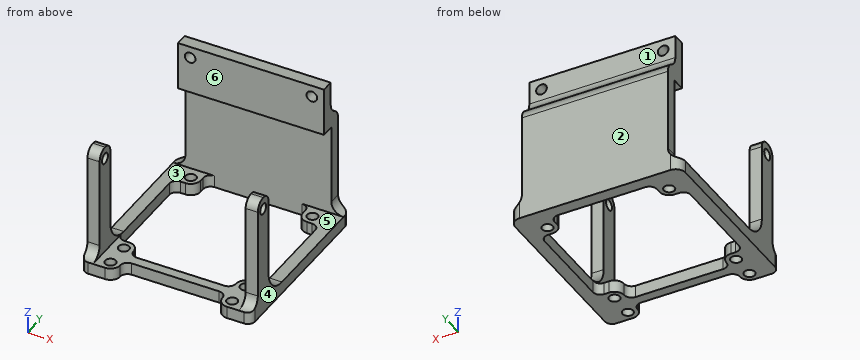
from build123d import *

# Parameters (mm, degrees)
SKETCH1_R           = 2.2
BOSS_EXTRUDE1_DEPTH = 5
FILLET1_R           = 3
FILLET2_R           = 3
SKETCH2_W           = 70
SKETCH2_H           = 43
BOSS_EXTRUDE2_DEPTH = 5
SKETCH3_W           = 70
SKETCH3_H           = 10.5
BOSS_EXTRUDE3_DEPTH = 5
SKETCH4_W           = 70
SKETCH4_H           = 5
BOSS_EXTRUDE4_DEPTH = 15
FILLET3_R           = 5.5
SKETCH6_W           = 5
SKETCH6_H           = 58
CUT_EXTRUDE1_DEPTH  = 15
FILLET4_R           = 5.5
FILLET5_R           = 5
SKETCH7_R           = 2.2
CUT_EXTRUDE2_DEPTH  = 15
SKETCH8_W           = 5
SKETCH8_H           = 8
BOSS_EXTRUDE5_DEPTH = 46
FILLET7_R           = 10
FILLET8_R           = 3
FILLET9_R           = 5
SKETCH10_R          = 2.2
CUT_EXTRUDE3_DEPTH  = 178.791001057
FILLET10_R          = 4
FILLET11_R          = 4
FILLET12_R          = 4


# Some blends are built 0.0001 mm under size
with BuildPart() as part:
    # Sketch1 → Boss-Extrude1 (new body)
    with BuildSketch(Plane.XY):
        with BuildLine():
            Line((-45.5, 87.8), (-45.5, 90.8))
            ThreePointArc((-45.5, 90.8), (-44.328427125, 93.628427125), (-41.5, 94.8))
            Line((-41.5, 94.8), (-36.5, 94.8))
            Line((-36.5, 94.8), (-36.5, 136.8))
            Line((-36.5, 136.8), (-41.5, 136.8))
            ThreePointArc((-41.5, 136.8), (-44.328427125, 137.971572875), (-45.5, 140.8))
            Line((-45.5, 140.8), (-45.5, 145.8))
            Line((-45.5, 145.8), (-36.5, 145.8))
            Line((-36.5, 145.8), (-31.5, 145.8))
            Line((-31.5, 145.8), (-31.5, 76.8))
            Line((-31.5, 76.8), (-36.5, 76.8))
            Line((-36.5, 76.8), (-41.5, 76.8))
            ThreePointArc((-41.5, 76.8), (-44.328427125, 77.971572875), (-45.5, 80.8))
            Line((-45.5, 80.8), (-45.5, 83.8))
            Line((-45.5, 83.8), (-87.5, 83.8))
            Line((-87.5, 83.8), (-87.5, 80.8))
            ThreePointArc((-87.5, 80.8), (-88.671572875, 77.971572875), (-91.5, 76.8))
            Line((-91.5, 76.8), (-96.5, 76.8))
            Line((-96.5, 76.8), (-101.5, 76.8))
            Line((-101.5, 76.8), (-101.5, 145.8))
            Line((-101.5, 145.8), (-96.5, 145.8))
            Line((-96.5, 145.8), (-87.5, 145.8))
            Line((-87.5, 145.8), (-87.5, 140.8))
            ThreePointArc((-87.5, 140.8), (-88.671572875, 137.971572875), (-91.5, 136.8))
            Line((-91.5, 136.8), (-96.5, 136.8))
            Line((-96.5, 136.8), (-96.5, 94.8))
            Line((-96.5, 94.8), (-91.5, 94.8))
            ThreePointArc((-91.5, 94.8), (-88.671572875, 93.628427125), (-87.5, 90.8))
            Line((-87.5, 90.8), (-87.5, 87.8))
            Line((-87.5, 87.8), (-45.5, 87.8))
        make_face()
        with Locations((-91.5, 140.8)):
            Circle(SKETCH1_R, mode=Mode.SUBTRACT)
        with Locations(Location((-41.5, 140.8, 0), (0, 0, 180))):
            Circle(SKETCH1_R, mode=Mode.SUBTRACT)
        with Locations((-41.5, 90.8)):
            Circle(SKETCH1_R, mode=Mode.SUBTRACT)
        with Locations(Location((-91.5, 90.8, 0), (0, 0, 180))):
            Circle(SKETCH1_R, mode=Mode.SUBTRACT)
        with Locations((-91.5, 80.8)):
            Circle(SKETCH1_R, mode=Mode.SUBTRACT)
        with Locations(Location((-41.5, 80.8, 0), (0, 0, 180))):
            Circle(SKETCH1_R, mode=Mode.SUBTRACT)
    extrude(amount=BOSS_EXTRUDE1_DEPTH)

    # Fillet1
    fillet1_edges = [part.edges().sort_by_distance(p)[0] for p in [
        (-36.5, 136.8, 2.5),
        (-96.5, 136.8, 2.5),
        (-36.5, 94.8, 2.5),
        (-45.5, 87.8, 2.5),
        (-45.5, 83.8, 2.5),
        (-87.5, 83.8, 2.5),
        (-87.5, 87.8, 2.5),
        (-96.5, 94.8, 2.5),
    ]]
    fillet(fillet1_edges, radius=FILLET1_R - 0.0001)  # a hair under: the kernel refuses the full size

    # Fillet2
    fillet2_edges = [part.edges().sort_by_distance(p)[0] for p in [
        (-31.5, 76.8, 2.5),
        (-101.5, 76.8, 2.5),
    ]]
    fillet(fillet2_edges, radius=FILLET2_R)

    # Sketch2 → Boss-Extrude2 (add)
    with BuildSketch(Plane(origin=(0, 145.8, 0), x_dir=(1, 0, 0), z_dir=(0, 1, 0))):
        with Locations((-66.5, -21.5)):
            Rectangle(SKETCH2_W, SKETCH2_H)
    extrude(amount=BOSS_EXTRUDE2_DEPTH)

    # Sketch3 → Boss-Extrude3 (add)
    with BuildSketch(Plane.XY.offset(43)):
        with Locations((-66.5, 145.55)):
            Rectangle(SKETCH3_W, SKETCH3_H)
    extrude(amount=BOSS_EXTRUDE3_DEPTH)

    # Sketch4 → Boss-Extrude4 (add)
    with BuildSketch(Plane.XY.offset(48)):
        with Locations((-66.5, 142.8)):
            Rectangle(SKETCH4_W, SKETCH4_H)
    extrude(amount=BOSS_EXTRUDE4_DEPTH)

    # Fillet3
    fillet3_edges = [part.edges().sort_by_distance(p)[0] for p in [
        (-66.5, 145.3, 48),
    ]]
    fillet(fillet3_edges, radius=FILLET3_R - 0.0001)  # a hair under: the kernel refuses the full size

    # Sketch6 → Cut-Extrude1 (cut)
    with BuildSketch(Plane(origin=(0, 150.8, 0), x_dir=(1, 0, 0), z_dir=(0, 1, 0))):
        with Locations((-99, -34)):
            Rectangle(SKETCH6_W, SKETCH6_H)
        with Locations((-34, -34)):
            Rectangle(SKETCH6_W, SKETCH6_H)
    extrude(amount=-CUT_EXTRUDE1_DEPTH, mode=Mode.SUBTRACT)

    # Fillet4
    fillet4_edges = [part.edges().sort_by_distance(p)[0] for p in [
        (-66.5, 150.8, 48),
    ]]
    fillet(fillet4_edges, radius=FILLET4_R)

    # Fillet5
    fillet5_edges = [part.edges().sort_by_distance(p)[0] for p in [
        (-36.5, 148.3, 5),
        (-96.5, 148.3, 5),
    ]]
    fillet(fillet5_edges, radius=FILLET5_R - 0.0001)  # a hair under: the kernel refuses the full size

    # Sketch7 → Cut-Extrude2 (cut)
    with BuildSketch(Plane(origin=(0, 145.3, 0), x_dir=(1, 0, 0), z_dir=(0, 1, 0))):
        with Locations(Location((-91.5, -58.25, 0), (0, 0, 270))):
            Circle(SKETCH7_R)
        with Locations(Location((-41.5, -58.25, 0), (0, 0, 270))):
            Circle(SKETCH7_R)
    extrude(amount=-CUT_EXTRUDE2_DEPTH, mode=Mode.SUBTRACT)

    # Sketch8 → Boss-Extrude5 (add)
    with BuildSketch(Plane.XY.offset(5)):
        with Locations((-99, 85.8)):
            Rectangle(SKETCH8_W, SKETCH8_H)
        with Locations((-34, 85.8)):
            Rectangle(SKETCH8_W, SKETCH8_H)
    extrude(amount=BOSS_EXTRUDE5_DEPTH)

    # Fillet7
    # the kernel refuses this fillet: 10 mm, written as the material it adds along each edge
    with BuildSketch(Plane(origin=(-101.5, 89.8, 5), x_dir=(0, 1, 0), z_dir=(1, 0, 0))) as fillet7_piece_1:
        with BuildLine():
            CenterArc((FILLET7_R, FILLET7_R), FILLET7_R, 180, 90)
            Line((0, FILLET7_R), (0, 0))
            Line((0, 0), (FILLET7_R, 0))
        make_face()
    extrude(amount=5)
    with BuildSketch(Plane(origin=(-31.5, 89.8, 5), x_dir=(0, 1, 0), z_dir=(-1, 0, 0))) as fillet7_piece_2:
        with BuildLine():
            CenterArc((FILLET7_R, -FILLET7_R), FILLET7_R, 90, 90)
            Line((0, -FILLET7_R), (0, 0))
            Line((0, 0), (FILLET7_R, 0))
        make_face()
    extrude(amount=5)

    # Fillet8
    fillet8_edges = [part.edges().sort_by_distance(p)[0] for p in [
        (-87.5, 145.8, 2.5),
        (-45.5, 145.8, 2.5),
    ]]
    fillet(fillet8_edges, radius=FILLET8_R)

    # Fillet9
    fillet9_edges = [part.edges().sort_by_distance(p)[0] for p in [
        (-34, 81.8, 5),
        (-99, 81.8, 5),
    ]]
    fillet(fillet9_edges, radius=FILLET9_R - 0.0001)  # a hair under: the kernel refuses the full size

    # Sketch10 → Cut-Extrude3 (cut, through all)
    with BuildSketch(Plane.ZY.offset(101.5)):
        with Locations((46, 85.8)):
            Circle(SKETCH10_R)
    extrude(amount=-CUT_EXTRUDE3_DEPTH, mode=Mode.SUBTRACT)

    # Fillet10
    fillet10_edges = [part.edges().sort_by_distance(p)[0] for p in [
        (-99, 81.8, 51),
        (-99, 89.8, 51),
        (-34, 81.8, 51),
        (-34, 89.8, 51),
    ]]
    fillet(fillet10_edges, radius=FILLET10_R - 0.0001)  # a hair under: the kernel refuses the full size

    # Fillet11
    fillet11_edges = [part.edges().sort_by_distance(p)[0] for p in [
        (-101.5, 150.8, 2.5),
    ]]
    fillet(fillet11_edges, radius=FILLET11_R)

    # Fillet12
    fillet12_edges = [part.edges().sort_by_distance(p)[0] for p in [
        (-31.5, 150.8, 2.5),
    ]]
    fillet(fillet12_edges, radius=FILLET12_R)


solid = part.part
Design review of the part built by this model. Coordinates are the model's own, in mm. Face numbers are marked on the shaded views. A direction names the side the tool comes from. Round coordinates to 2 decimals unless told otherwise and drop trailing zeros. Write each loop counter-clockwise with the first axis right and the second up, starting at its lowest first coordinate (ties: lowest second). Pieces come first, ordered by that corner, then holes. Notation, with made-up numbers: M 74.25,87.25 L 99.25,87.25 A22 ccw 99.25,97.25 Z; hole C -39,42 d4. An arc over 180 degrees is marked long. One line per item, written item: value. Start each with the question number.
1. For the marked faces 1, 2 and 3, list the 3-axis set-ups (+Z, -Z, +X, -X, +Y, -Y) from which the entire face can be reached by the end or side of a thin tool; tool diameter is ignored.
2. Clearance check with flat-ended pins moving along their axes: P1, Ø16, axis at x = -57.5, z = 51, coming from the -Y side; P2, Ø4, axis at x = -61.5, z = 55, coming from the +Y side; P3, Ø5, axis at x = -51, z = 22.5, coming from the -Y side. State where each tip first meets the part, or that it passes through.
3. Take a section at B-B on z = 26. State the section outline as (x, y) points, then the cut area to 3 significant figures.
4. Take a section at A-A on z = 58.25. State the section outline as (x, y) points, then the cut area to 3 significant figures.
5. To check wall thickness, follow probe 1 along X at (y, z) = (140.8, 1.1); probe 2 along X at (y, z) = (140, 1); probe 3 along Z at (x, y) = (-93, 94.5). State the ranges of each line that lie inside material, in increasing order. Write a range as from..to.
6. Draft analysis for pull direction Y (two halves, no side actions). For the marked faces 4, 5 and 6, state which applies: pulls with the +Y half, pulls with the -Y half, needs draft (parallel to the pull), parting line crosses it, or undercut.
Computed:
1. face 1: +Z, +X, -X, +Y
1. face 2: +Z, -Z, +X, -X, +Y
1. face 3: +X, -X
2. P1: stops at y = 140.3
2. P2: stops at y = 145.32
2. P3: stops at y = 145.8
3. outline: M -101.5,81.8 L -96.5,81.8 L -96.5,89.8 L -101.5,89.8 Z; M -96.5,145.8 L -36.5,145.8 L -36.5,150.8 L -96.5,150.8 Z; M -36.5,81.8 L -31.5,81.8 L -31.5,89.8 L -36.5,89.8 Z
3. area: 380 mm²
4. outline: M -96.5,140.3 L -93.7,140.3 L -93.7,145.3 L -96.5,145.3 Z; M -89.3,140.3 L -43.7,140.3 L -43.7,145.3 L -89.3,145.3 Z; M -39.3,140.3 L -36.5,140.3 L -36.5,145.3 L -39.3,145.3 Z
4. area: 256 mm²
5. probe 1: x = -101.5..-93.7, -89.3..-87.5, -45.5..-43.7, -39.3..-31.5
5. probe 2: x = -101.5..-93.55, -89.45..-87.58, -45.42..-43.55, -39.45..-31.5
5. probe 3: z = 0..5
6. face 4: needs draft
6. face 5: undercut
6. face 6: pulls with the -Y half
